```python
from build123d import *

# Parameters (mm, degrees)
SKETCH_1_W          = 60
SKETCH_1_H          = 30
EXTRUDE_1_DEPTH     = 10
SKETCH_2_R          = 2.9
EXTRUDE_2_DEPTH     = 9.8
EXTRUDE_START       = -9.8
SKETCH_4_R          = 2.9
EXTRUDE_3_DEPTH     = 9.8
SKETCH_5_R          = 2.4
CUT_EXTRUDE_1_DEPTH = 6
CUT_EXTRUDE_2_DEPTH = 4.2
CUT_EXTRUDE_3_DEPTH = 2.4
SKETCH_8_R          = 2.4
CUT_EXTRUDE_4_DEPTH = 47.983082062
FILLET_1_R          = 1
FILLET_2_R          = 2
CHAMFER_5_SIZE      = 1


with BuildPart() as part:
    # 草圖1 → 填料-伸長1 (new body)
    with BuildSketch(Plane(origin=(0, 0, 0), x_dir=(1, 0, 0), z_dir=(0, 1, 0))):
        Rectangle(SKETCH_1_W, SKETCH_1_H)
    extrude(amount=EXTRUDE_1_DEPTH)

    # 草圖2 → 填料-伸長2 (add)
    with BuildSketch(Plane.XY.offset(15)):
        with BuildLine():
            Line((-9.836356149, 35.713371359), (-30, 10))
            Line((-30, 10), (30, 10))
            Line((30, 10), (9.836356149, 35.713371359))
            ThreePointArc((9.836356149, 35.713371359), (0, 40.5), (-9.836356149, 35.713371359))
        make_face()
        with Locations((0, 28)):
            Circle(SKETCH_2_R, mode=Mode.SUBTRACT)
    extrude(amount=-EXTRUDE_2_DEPTH)

    # 草圖4 → 填料-伸長3 (add)
    with BuildSketch(Plane(origin=(0, 0, -15), x_dir=(-1, 0, 0), z_dir=(0, 0, -1)).offset(EXTRUDE_START)):
        with BuildLine():
            Line((30, 10), (9.836356149, 35.713371359))
            ThreePointArc((9.836356149, 35.713371359), (0, 40.5), (-9.836356149, 35.713371359))
            Line((-9.836356149, 35.713371359), (-30, 10))
            Line((-30, 10), (30, 10))
        make_face()
        with Locations(Location((0, 28, 0), (0, 0, 180))):
            Circle(SKETCH_4_R, mode=Mode.SUBTRACT)
    extrude(amount=EXTRUDE_3_DEPTH)

    # 草圖5 → 除料-伸長1 (cut)
    with BuildSketch(Plane.XZ):
        with Locations(Location((20, 10, 0), (0, 0, 270))):
            Circle(SKETCH_5_R)
        with Locations(Location((20, -10, 0), (0, 0, 270))):
            Circle(SKETCH_5_R)
        with Locations(Location((-20, -10, 0), (0, 0, 270))):
            Circle(SKETCH_5_R)
        with Locations(Location((-20, 10, 0), (0, 0, 270))):
            Circle(SKETCH_5_R)
    extrude(amount=-CUT_EXTRUDE_1_DEPTH, mode=Mode.SUBTRACT)

    # 草圖6 → 除料-伸長2 (cut)
    with BuildSketch(Plane.XY.offset(15)):
        Polygon((0, 32.618802154), (-4, 30.309401077), (-4, 25.690598923), (0, 23.381197846), (4, 25.690598923), (4, 30.309401077), align=None)
    extrude(amount=-CUT_EXTRUDE_2_DEPTH, mode=Mode.SUBTRACT)

    # 草圖7 → 除料-伸長3 (cut)
    with BuildSketch(Plane(origin=(0, 10, 0), x_dir=(1, 0, 0), z_dir=(0, 1, 0))):
        Polygon((3.175426481, 0), (1.58771324, 2.75), (-1.58771324, 2.75), (-3.175426481, 0), (-1.58771324, -2.75), (1.58771324, -2.75), align=None)
    extrude(amount=-CUT_EXTRUDE_3_DEPTH, mode=Mode.SUBTRACT)

    # 草圖8 → 除料-伸長4 (cut, through all)
    with BuildSketch(Plane(origin=(0, 7.6, 0), x_dir=(1, 0, 0), z_dir=(0, 1, 0))):
        with Locations(Location((0, 0, 0), (0, 0, 270))):
            Circle(SKETCH_8_R)
    extrude(amount=-CUT_EXTRUDE_4_DEPTH, mode=Mode.SUBTRACT)

    # 圓角1
    fillet_1_edges = [part.edges().sort_by_distance(p)[0] for p in [
        (-19.918178074, 22.856685679, 5.2),
        (0, 40.5, 5.2),
        (19.918178074, 22.856685679, 5.2),
        (0, 40.5, -5.2),
        (-19.918178074, 22.856685679, -5.2),
        (19.918178074, 22.856685679, -5.2),
    ]]
    fillet(fillet_1_edges, radius=FILLET_1_R)

    # 圓角2
    fillet_2_edges = [part.edges().sort_by_distance(p)[0] for p in [
        (19.918178074, 22.856685679, 15),
        (0, 40.5, 15),
        (-19.918178074, 22.856685679, 15),
        (0, 40.5, -15),
        (19.918178074, 22.856685679, -15),
        (-19.918178074, 22.856685679, -15),
        (30, 5, 15),
        (-30, 5, 15),
        (-30, 5, -15),
        (30, 5, -15),
    ]]
    fillet(fillet_2_edges, radius=FILLET_2_R)

    # 導角5
    chamfer_5_edges = [part.edges().sort_by_distance(p)[0] for p in [
        (2.38156986, 10, 1.375),
        (2.38156986, 10, -1.375),
        (0, 10, -2.75),
        (-2.38156986, 10, -1.375),
        (-2.38156986, 10, 1.375),
        (0, 10, 2.75),
    ]]
    chamfer(chamfer_5_edges, length=CHAMFER_5_SIZE)


solid = part.part
```
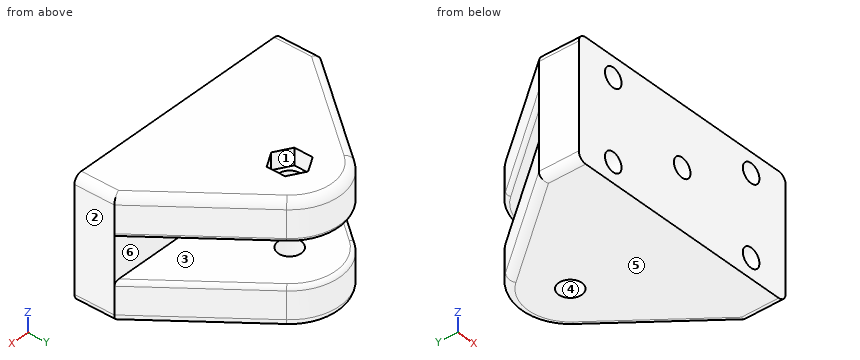
Design review of the part built by this model. Coordinates are the model's own, in mm. Face numbers are marked on the shaded views. A direction names the side the tool comes from. Give positions to 0.01 mm unless a question says otherwise; leave off trailing zeros. Order: outer loops, then holes, each group sorted by start corner. A loop starts at its lowest first (then second) coordinate and runs counter-clockwise, first axis right, second up. Notation, with made-up numbers: (-20.75, -5.5) - (8.25, -5.5) arc R21 ccw to (8.25, 26.5) - close; hole circle Ø3 at (-22, 73). An arc over 180 degrees is marked (long way). Use a Markdown table: item, result. Add a question column.
(1) Clearance check with flat-ended pins moving along their axes: P1, Ø5, axis at x = -6.5, z = 10.5, coming from the +Y side; P2, Ø4, axis at x = -20, z = 10, coming from the +Y side; P3, Ø4, axis at x = 4.5, z = 7.5, coming from the +Y side. State where each tip first meets the part, or that it passes through.
(2) Add section B-B on y = 28. Give the number of separate pieces and of enclosed holes in the cut face, then the cut area to 3 significant figures.
(3) Wall thickness on probe 1 along X at (y, z) = (4.8, -10); probe 2 along Z at (x, y) = (14, 24); probe 3 along Y at (x, z) = (0, -7.25): over which ranges is each line inside the solid? List them lowest first. Write a range as [from, to].
(4) Add section C-C on z = -10.75. Give the boundary of the cut face in (x, y), then the cut area to 3 significant figures.
(5) Add section A-A on z = 10. Give the boundary of the cut face in (x, y), then the cut area to 3 significant figures.
(6) Mouldability with a two-part tool opening along Z and no side actions: class the marked faces 3, 4, 5 and 6 as +Z half, -Z half, draft (parallel to the pull), parting line (faces both ways), or undercut.
(7) Machinability: for the marked faces 1 and 2, which of the approach directions +Z, -Z, +X, -X, +Y, -Y give a long, thin tool a straight path to every point of the face, cutting with its end or side? Answer none if there is none.
Report:
| question | item | result |
|---|---|---|
| 1 | P1 | stops at y = 39.84 |
| 1 | P2 | stops at y = 25.3 |
| 1 | P3 | stops at y = 40.25 |
| 2 | separate pieces | 4 |
| 2 | enclosed holes | 0 |
| 2 | area | 494 mm² |
| 3 | probe 1 | x = [-30, -22.4], [-17.6, 17.6], [22.4, 30] |
| 3 | probe 2 | z = [-15, -5.2], [5.2, 15] |
| 3 | probe 3 | y = [0, 25.1], [30.9, 40.5] |
| 4 | outline | (-30, 0) - (-22.28, 0) - (-22.28, 6) - (-17.72, 6) - (-17.72, 0) - (17.72, 0) - (17.72, 6) - (22.28, 6) - (22.28, 0) - (30, 0) - (30, 10) - (9.84, 35.71) arc R12.5 ccw to (-9.84, 35.71) - (-30, 10) - close; hole circle Ø5.8 at (0, 28) |
| 4 | area | 1,610 mm² |
| 5 | outline | (-30, 0) - (-22.4, 0) - (-22.4, 6) - (-17.6, 6) - (-17.6, 0) - (17.6, 0) - (17.6, 6) - (22.4, 6) - (22.4, 0) - (30, 0) - (30, 10) - (9.84, 35.71) arc R12.5 ccw to (-9.84, 35.71) - (-30, 10) - close; hole circle Ø5.8 at (0, 28) |
| 5 | area | 1,610 mm² |
| 6 | face 3 | undercut |
| 6 | face 4 | draft |
| 6 | face 5 | -Z half |
| 6 | face 6 | undercut |
| 7 | face 1 | +Z |
| 7 | face 2 | +Z, -Z, +X, +Y, -Y |
